Part print with two shaded views. Sizes in mm from the minimum x, y, z corner. A direction names the side the tool comes from. Round coordinates to 2 decimals unless told otherwise and drop trailing zeros. Loops run counter-clockwise (first coordinate to the right, second up) from the corner with the lowest first, then second, coordinate; pieces in that order, holes last. Notation, with made-up numbers: (50, 21.5) - (89, 21.5) arc R18 ccw to (89, 42.5) - close; hole circle Ø10 at (-1, 31). An arc over 180 degrees is marked (long way). One line per question, with ' | ' between items.
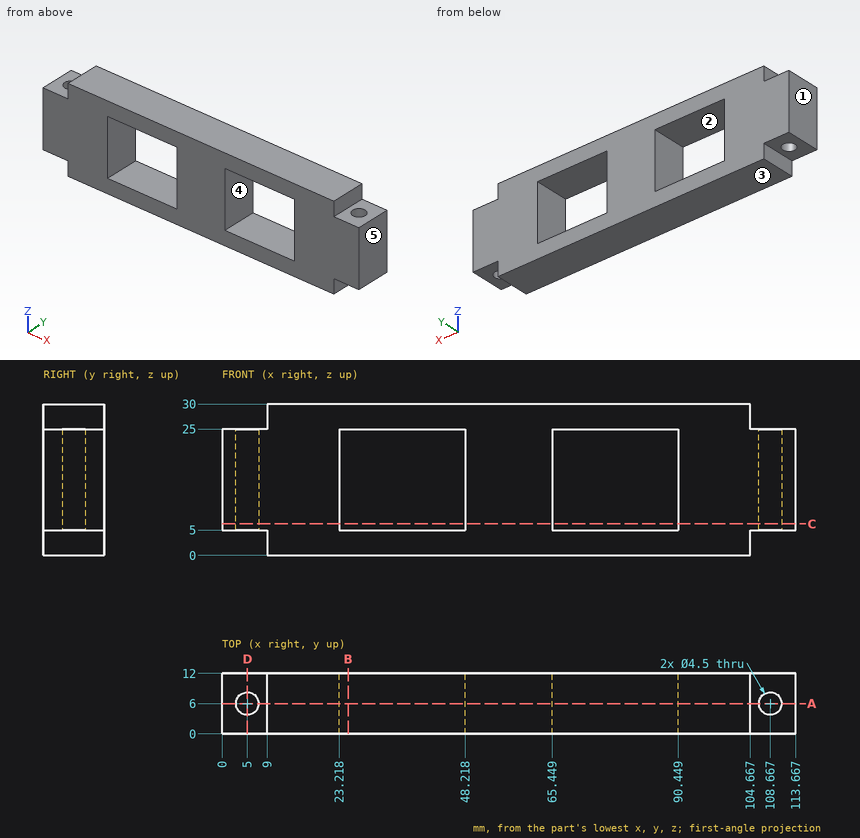
(1) Cut at B-B, the plane x = 25. Write the cut outline in (y, z).
Results found:
outline: (0, 0) - (12, 0) - (12, 5) - (0, 5) - close; (0, 25) - (12, 25) - (12, 30) - (0, 30) - close
(2) Drop flat-ended pins along their axis: P1, Ø1.5, axis at y = 8.5, z = 3, coming from the -X side; P2, Ø2.5, axis at y = 6.5, z = 26.5, coming from the +X side; P3, Ø4.5, axis at x = 2.5, y = 6, coming from the -Z side. Give the stop position or say it passes through.
Results found:
P1: stops at x = 9 | P2: stops at x = 104.67 | P3: stops at z = 5
(3) Cut at A-A, the plane y = 6. Write the cut outline in (x, z), then the cut area to 3 significant figures.
Results found:
outline: (0, 5) - (2.75, 5) - (2.75, 25) - (0, 25) - close; (7.25, 5) - (9, 5) - (9, 0) - (104.67, 0) - (104.67, 5) - (106.42, 5) - (106.42, 25) - (104.67, 25) - (104.67, 30) - (9, 30) - (9, 25) - (7.25, 25) - close; (110.92, 5) - (113.67, 5) - (113.67, 25) - (110.92, 25) - close; hole (23.22, 5) - (48.22, 5) - (48.22, 25) - (23.22, 25) - close; hole (65.45, 5) - (90.45, 5) - (90.45, 25) - (65.45, 25) - close | area: 2,050 mm²
(4) Two-plate mould, pull along X, no slides. Class the marked faces 3, 4 and 5: released by +X, released by -X, zero draft, split by the parting line, or undercut.
Results found:
face 3: zero draft | face 4: undercut | face 5: released by +X
(5) Tool access for the marked faces 1 and 2: list every direction of +Z, -Z, +X, -X, +Y, -Y with a clear straight run to the whole face (end or side of a thin tool).
Results found:
face 1: +Z, -Z, -X, +Y, -Y | face 2: +Y, -Y
(6) Cut at C-C, the plane z = 6.25. Write the cut outline in (x, y), then the cut area to 3 significant figures.
Results found:
outline: (0, 0) - (23.22, 0) - (23.22, 12) - (0, 12) - close; (48.22, 0) - (65.45, 0) - (65.45, 12) - (48.22, 12) - close; (90.45, 0) - (113.67, 0) - (113.67, 12) - (90.45, 12) - close; hole circle Ø4.5 at (5, 6); hole circle Ø4.5 at (108.67, 6) | area: 732 mm²
(7) Probe L1, parallel to X at y = 10.75, z = 7.5; L2, parallel to X at y = 5.75, z = 23.75; L3, parallel to Z at x = 72, y = 1.5. List the from-to ranges inside material, lowest first.
Results found:
L1: x = 0 to 23.22, 48.22 to 65.45, 90.45 to 113.67 | L2: x = 0 to 2.76, 7.24 to 23.22, 48.22 to 65.45, 90.45 to 106.43, 110.9 to 113.67 | L3: z = 0 to 5, 25 to 30
(8) Cut at D-D, the plane x = 5. Write the cut outline in (y, z), then the cut area to 3 significant figures.
Results found:
outline: (0, 5) - (3.75, 5) - (3.75, 25) - (0, 25) - close; (8.25, 5) - (12, 5) - (12, 25) - (8.25, 25) - close | area: 150 mm²
